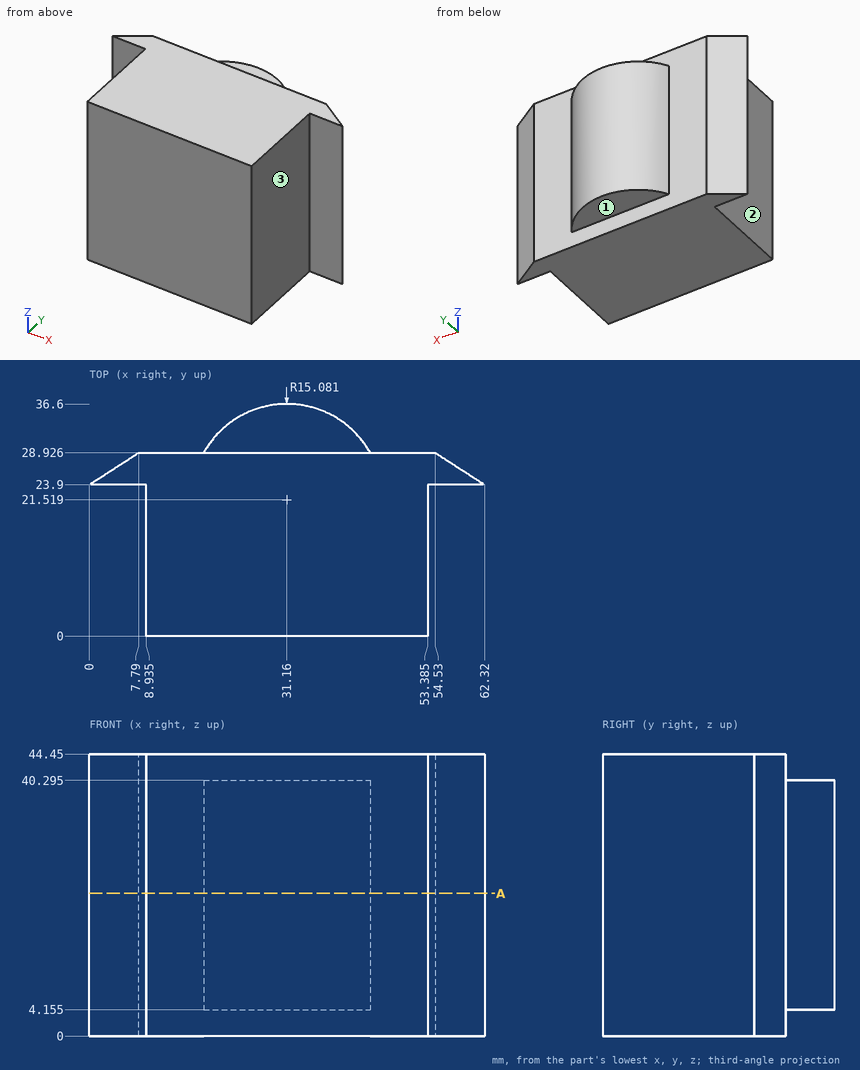
Here's the drawing with two shaded views (mm, measured from the low corner). I have some questions. A direction names the side the tool comes from. Coordinates: 2 decimals unless noted, no trailing zeros. Order: outer loops, then holes, each group sorted by start corner. A loop starts at its lowest first (then second) coordinate and runs counter-clockwise, first axis right, second up.
Item 1: If we section it at A-A, the plane z = 22.5: List the corners of the cut face in (x, y) for me (1 decimal).
Response values:
outline: (0, 23.9) - (8.9, 23.9) - (8.9, 0) - (53.4, 0) - (53.4, 23.9) - (62.3, 23.9) - (54.5, 28.9) - (44.3, 28.9) arc R15.1 ccw to (18, 28.9) - (7.8, 28.9) - close
Item 2: I need wall thicknesses on probe 1 along X at (y, z) = (18, 22.5) (1 decimal); probe 2 along Y at (x, z) = (20.5, 2) (1 decimal); probe 3 along Z at (x, y) = (41, 32.5) (1 decimal). Which ranges of each line are inside material? Lowest first, please.
Response values:
probe 1: x = 8.9 to 53.4
probe 2: y = 0 to 28.9
probe 3: z = 4.2 to 40.3
Item 3: I'm going to push flat-ended pins straight in: pin 1 Ø6 at (x, z) = (7.5, 35.5) entering from +Y; pin 2 Ø1.5 at (y, z) = (27.5, 24.5) entering from -X; pin 3 Ø10 at (y, z) = (7.5, 20) entering from -X (1 decimal). Where does each tip first touch, or does it pass through?
Response values:
pin 1: stops at y = 28.93
pin 2: stops at x = 4.42
pin 3: stops at x = 8.9
Item 4: Which directions (+Z, -Z, +X, -X, +Y, -Y) give clear straight access to the entire face, cutting with the end or side of a thin tool? Please do the marked faces 1, 2 and 3.
Response values:
face 1: -Z, +X, -X, +Y
face 2: +Z, -Z, -X, -Y
face 3: +Z, -Z, +X, -Y
